```python
from build123d import *

# Parameters (mm, degrees)
SKETCH1_R           = 2.975
BOSS_EXTRUDE1_DEPTH = 4.9
BOSS_EXTRUDE2_START = -1
SKETCH2_R           = 2.975
BOSS_EXTRUDE2_DEPTH = 1


with BuildPart() as part:
    # Sketch1 → Boss-Extrude1 (new body)
    with BuildSketch(Plane.XY):
        Circle(SKETCH1_R)
        with BuildLine():
            Line((-1.118033989, 1), (1.118033989, 1))
            ThreePointArc((1.118033989, 1), (0, -1.5), (-1.118033989, 1))
        make_face(mode=Mode.SUBTRACT)
    extrude(amount=BOSS_EXTRUDE1_DEPTH)

    # Sketch2 → Boss-Extrude2 (add)
    with BuildSketch(Plane.XY.offset(4.9).offset(BOSS_EXTRUDE2_START)):
        with BuildLine():
            Line((3.4, -2.059277786), (3.4, 2.059277786))
            ThreePointArc((3.4, 2.059277786), (0, 3.975), (-3.4, 2.059277786))
            Line((-3.4, 2.059277786), (-3.4, -2.059277786))
            ThreePointArc((-3.4, -2.059277786), (0, -3.975), (3.4, -2.059277786))
        make_face()
        Circle(SKETCH2_R, mode=Mode.SUBTRACT)
    extrude(amount=BOSS_EXTRUDE2_DEPTH)


solid = part.part
```
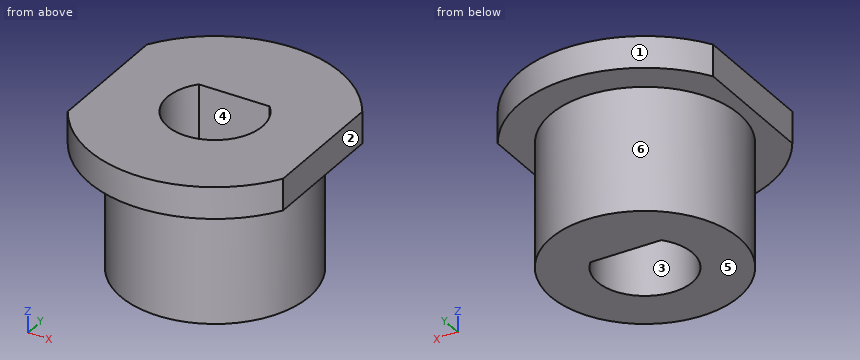
Can you work these out from the model? Positions are in its coordinate system, mm. Face numbers are marked on the shaded views. A direction names the side the tool comes from. Round coordinates to 2 decimals unless told otherwise and drop trailing zeros. Loops run counter-clockwise (first coordinate to the right, second up) from the corner with the lowest first, then second, coordinate; pieces in that order, holes last. Notation, with made-up numbers: M -18.75,-18.75 L 13.25,-18.75 A7 cw 13.25,-6.75 Z; hole C 56.5,27.25 d6. An arc over 180 degrees is marked long. Answer as a JSON object with one key per item and string values. Group by question number.
Q1. Please list where these lines run through material, in increasing order: L1, parallel to Z at x = -0.75, y = 3.25; L2, parallel to X at y = 0.5, z = 4.65; L3, parallel to Y at x = 0.25, z = 3.8.
Q2. Imagine slicing it at D-D, the plane y = 1.5. Please give me the cut outline in (x, z), then the cut area to 3 significant figures.
Q3. Imagine slicing it at C-C, the plane z = 1.45. Please give me the cut outline in (x, y) (3 decimals).
Q4. Will these pins go through, and if not, where does the flat tip stop? pin 1 (1.5 mm diameter, centred on x = 2.5, y = -3, fed in from -Z); pin 2 (2 mm diameter, centred on x = 1, z = 2, fed in from -Y) (3 decimals).
Q5. Imagine slicing it at A-A, the plane y = 0. Please give me the cut outline in (x, z) (3 decimals).
Q6. Imagine slicing it at B-B, the plane x = 0.75. Please give me the cut outline in (y, z), then the cut area to 3 significant figures.
Q7. On a 3-axis mill with a long thin cutter (end or side, diameter ignored), from which of +Z, -Z, +X, -X, +Y, -Y can I reach the whole of each face in a straight line? I mean the marked faces 5 and 6. Say none if no direction works.
Q8. We'd pull the mould along X, two halves only. Please class the marked faces 1, 2, 3 and 4: +X half, -X half, draft (parallel to the pull), parting line (faces both ways), or undercut.
Findings:
{
 "1": {"L1": "z = 3.9 to 4.9", "L2": "x = -3.4 to -1.41, 1.41 to 3.4", "L3": "y = -2.96 to -1.48, 1 to 2.96"},
 "2": {"outline": "M -3.4,3.9 L -2.57,3.9 L -2.57,0 L 2.57,0 L 2.57,3.9 L 3.4,3.9 L 3.4,4.9 L -3.4,4.9 Z", "area": "26.8 mm2"},
 "3": {"outline": "C 0,0 d5.95; hole M -1.118,1 A1.5 ccw long 1.118,1 Z"},
 "4": {"pin 1": "stops at z = 3.9", "pin 2": "stops at y = -2.975"},
 "5": {"outline": "M -3.4,3.9 L -2.975,3.9 L -2.975,0 L -1.5,0 L -1.5,4.9 L -3.4,4.9 Z; M 1.5,0 L 2.975,0 L 2.975,3.9 L 3.4,3.9 L 3.4,4.9 L 1.5,4.9 Z"},
 "6": {"outline": "M -3.9,3.9 L -2.88,3.9 L -2.88,0 L -1.3,0 L -1.3,4.9 L -3.9,4.9 Z; M 1,0 L 2.88,0 L 2.88,3.9 L 3.9,3.9 L 3.9,4.9 L 1,4.9 Z", "area": "19.0 mm2"},
 "7": {"face 5": "-Z, +X, -X, +Y, -Y", "face 6": "-Z"},
 "8": {"face 1": "parting line", "face 2": "+X half", "face 3": "undercut", "face 4": "undercut"}
}
